from build123d import *

# Parameters (mm, degrees)
SKETCH1_R             = 2.6
BOSS_EXTRUDE1_DEPTH   = 1.6
SKETCH2_R             = 3.45
BOSS_EXTRUDE2_DEPTH   = 1.4
M5X0_8_TAPPED_HOLE1_D = 4.2


with BuildPart() as part:
    # Sketch1 → Boss-Extrude1 (new body)
    with BuildSketch(Plane.XY):
        with BuildLine():
            Line((-10, -8.5), (-10, -5))
            Line((-10, -5), (-37.5, -5))
            Line((-37.5, -5), (-40.974341649, -3.841886117))
            ThreePointArc((-40.974341649, -3.841886117), (-41.716863278, -3.295926597), (-42, -2.41886117))
            Line((-42, -2.41886117), (-42, 2.41886117))
            ThreePointArc((-42, 2.41886117), (-41.716863278, 3.295926597), (-40.974341649, 3.841886117))
            Line((-40.974341649, 3.841886117), (-37.5, 5))
            Line((-37.5, 5), (-10, 5))
            Line((-10, 5), (-10, 8.5))
            ThreePointArc((-10, 8.5), (-9.560660172, 9.560660172), (-8.5, 10))
            Line((-8.5, 10), (-5, 10))
            Line((-5, 10), (-5, 37.5))
            Line((-5, 37.5), (-3.841886117, 40.974341649))
            ThreePointArc((-3.841886117, 40.974341649), (-3.295926597, 41.716863278), (-2.41886117, 42))
            Line((-2.41886117, 42), (2.41886117, 42))
            ThreePointArc((2.41886117, 42), (3.295926597, 41.716863278), (3.841886117, 40.974341649))
            Line((3.841886117, 40.974341649), (5, 37.5))
            Line((5, 37.5), (5, 10))
            Line((5, 10), (8.5, 10))
            ThreePointArc((8.5, 10), (9.560660172, 9.560660172), (10, 8.5))
            Line((10, 8.5), (10, -8.5))
            ThreePointArc((10, -8.5), (9.560660172, -9.560660172), (8.5, -10))
            Line((8.5, -10), (5, -10))
            Line((5, -10), (-5, -10))
            Line((-5, -10), (-8.5, -10))
            ThreePointArc((-8.5, -10), (-9.560660172, -9.560660172), (-10, -8.5))
        make_face()
        Circle(SKETCH1_R, mode=Mode.SUBTRACT)
    extrude(amount=BOSS_EXTRUDE1_DEPTH)

    # Sketch2 → Boss-Extrude2 (add)
    with BuildSketch(Plane.XY.offset(1.6)):
        with Locations((0, 14.95)):
            Circle(SKETCH2_R)
        with Locations((0, 34.95)):
            Circle(SKETCH2_R)
        with Locations((-14.95, 0)):
            Circle(SKETCH2_R)
        with Locations((-34.95, 0)):
            Circle(SKETCH2_R)
    extrude(amount=BOSS_EXTRUDE2_DEPTH)

    # M5x0.8 Tapped Hole1 (through all)
    with Locations(Plane.XY.offset(3)):
        with Locations((0, 34.95), (0, 14.95), (-14.95, 0), (-34.95, 0)):
            Hole(M5X0_8_TAPPED_HOLE1_D / 2)


solid = part.part
Design review of the part built by this model. Coordinates are the model's own, in mm. A direction names the side the tool comes from. Round coordinates to 2 decimals unless told otherwise and drop trailing zeros. Write each loop counter-clockwise with the first axis right and the second up, starting at its lowest first coordinate (ties: lowest second). Pieces come first, ordered by that corner, then holes. Notation, with made-up numbers: (-36.5, 37.5) - (-31.5, 37.5) arc R26 cw to (-31.5, 76.5) - close; hole circle Ø10 at (-27.75, 9.25). An arc over 180 degrees is marked (long way). Return JSON: item names as keys, results as strings. Group by question number.
Item 1: Insertion check: P1, Ø0.5, axis at y = 28, z = 0.5, coming from the +X side; P2, Ø1.3, axis at x = -7, z = 1, coming from the +Y side; P3, Ø5, axis at x = -34.95, y = 0, coming from the +Z side; P4, Ø1, axis at y = 35.5, z = 2.5, coming from the +X side. Each pin has a flat end and moves straight along its axis. Give the tip position at first contact, or say it passes through.
Item 2: We need section A-A on z = 2.1. Write out the cut boundary in (x, y), and give its area (3 significant figures).
Item 3: We need section B-B on x = -34.95. Write out the cut boundary in (y, z).
Item 4: For probe 1 along Y at (x, z) = (0, 1.45); probe 2 along Y at (x, z) = (-34.95, 1.7); probe 3 along Y at (x, z) = (-14.95, 1.2), list the stretches that pass through material, from the lowest coordinate up. Write a range as [from, to].
Item 5: Machinability: for faces 4 (the face through (-6, 6, 1.6)), 5 (the face through (-5, 24, 1)), 6 (the face through (-39.21, -4.43, 0.79)), which of the approach directions +Z, -Z, +X, -X, +Y, -Y give a long, thin tool a straight path to every point of the face, cutting with its end or side? Answer none if there is none.
Item 6: We need section D-D on y = 0. Write out the cut boundary in (x, z).
Item 7: The part is to be moulded in two halves that separate along X. For faces 1 (the face through (3.29, 41.72, 0.79)), 2 (the face through (-38.397, 0.152, 2.29)), 3 (the face through (-24, 5, 1)), say which applies: pulls with the +X half, pulls with the -X half, needs draft (parallel to the pull), parting line crosses it, or undercut.
Model answer:
{
 "1": {"P1": "stops at x = 5", "P2": "stops at y = 10", "P3": "stops at z = 3", "P4": "stops at x = 3.45"},
 "2": {"outline": "circle Ø6.9 at (-34.95, 0); circle Ø6.9 at (-14.95, 0); circle Ø6.9 at (0, 14.95); circle Ø6.9 at (0, 34.95); hole circle Ø4.2 at (-34.95, 0); hole circle Ø4.2 at (-14.95, 0); hole circle Ø4.2 at (0, 14.95); hole circle Ø4.2 at (0, 34.95)", "area": "94.2 mm²"},
 "3": {"outline": "(-5, 0) - (-2.1, 0) - (-2.1, 3) - (-3.45, 3) - (-3.45, 1.6) - (-5, 1.6) - close; (2.1, 0) - (5, 0) - (5, 1.6) - (3.45, 1.6) - (3.45, 3) - (2.1, 3) - close"},
 "4": {"probe 1": "y = [-10, -2.6], [2.6, 12.85], [17.05, 32.85], [37.05, 42]", "probe 2": "y = [-3.45, -2.1], [2.1, 3.45]", "probe 3": "y = [-5, -2.1], [2.1, 5]"},
 "5": {"face 4": "+Z", "face 5": "+Z, -Z, -X, +Y", "face 6": "+Z, -Z, -X, -Y"},
 "6": {"outline": "(-42, 0) - (-37.05, 0) - (-37.05, 3) - (-38.4, 3) - (-38.4, 1.6) - (-42, 1.6) - close; (-32.85, 0) - (-17.05, 0) - (-17.05, 3) - (-18.4, 3) - (-18.4, 1.6) - (-31.5, 1.6) - (-31.5, 3) - (-32.85, 3) - close; (-12.85, 0) - (-2.6, 0) - (-2.6, 1.6) - (-11.5, 1.6) - (-11.5, 3) - (-12.85, 3) - close; (2.6, 0) - (10, 0) - (10, 1.6) - (2.6, 1.6) - close"},
 "7": {"face 1": "pulls with the +X half", "face 2": "undercut", "face 3": "needs draft"}
}
